The listing builds one solid part. Answer for the finished solid, in the listing's coordinates (mm). Coordinates: 2 decimals unless noted, no trailing zeros. Order: outer loops, then holes, each group sorted by start corner. A loop starts at its lowest first (then second) coordinate and runs counter-clockwise, first axis right, second up. Notation, with made-up numbers: (9.5, 8.5) -> (47.5, 8.5) arc R35 cw to (47.5, 47.5) -> close; hole circle Ø9 at (81.5, -32.5). An arc over 180 degrees is marked (long way). Answer in a Markdown table with one row per item. Add a question column.
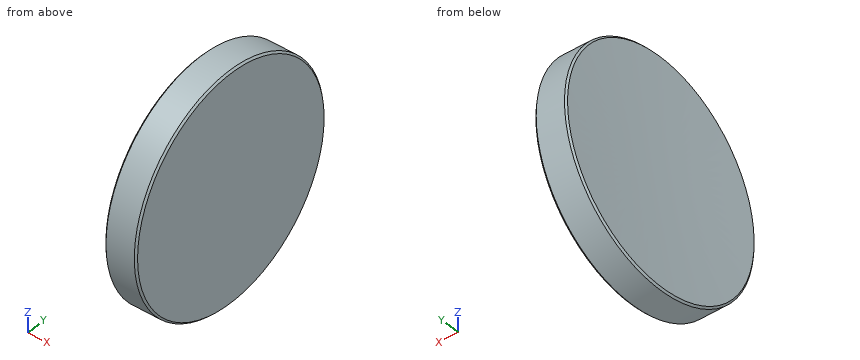
```python
from build123d import *

# Parameters (mm, degrees)
CHAMFER_1_SIZE2       = 0.25
CHAMFER_1_SIZE        = 0.237681877
CHAMFER_1_EDGE_2_SIZE = 0.25


with BuildPart() as part:
    # Эскиз1 → Повернуть1 (revolve)
    with BuildSketch(Plane.XY):
        with BuildLine():
            Line((-0.426259063, 16), (4, 16))
            Line((4, 16), (4, 0))
            Line((4, 0), (0, 0))
            ThreePointArc((0, 0), (-0.106583668, 8.002838509), (-0.426259063, 16))
        make_face()
    revolve(axis=Axis((4, 0, 0), (-1, 0, 0)))

    # Фаска1
    chamfer_1_edges = [part.edges().sort_by_distance(p)[0] for p in [
        (-0.426259063, -16, 0),
    ]]
    chamfer(chamfer_1_edges, length=CHAMFER_1_SIZE, length2=CHAMFER_1_SIZE2)

    # Фаска1 edge 2
    chamfer_1_edge_2_edges = [part.edges().sort_by_distance(p)[0] for p in [
        (4, -16, 0),
    ]]
    chamfer(chamfer_1_edge_2_edges, length=CHAMFER_1_EDGE_2_SIZE)


solid = part.part
```
Q1. Straight lines are drawn through the part: line 1 (X direction, y = -8, z = 6.5); line 2 (Y direction, x = 1.3, z = -3); line 3 (Y direction, x = 2.8, z = -7.5). For each, find the intervals that lie inside material, in ascending order.
Q2. Given pin 1 (1 mm diameter, centred on x = 2, z = -3.5, fed in from +Y); pin 2 (2 mm diameter, centred on x = 3, z = -11, fed in from +Y); pin 3 (1.5 mm diameter, centred on x = 2.5, y = -11, fed in from +Z), each flat-ended and moving along its own axis, determine where each tip first touches the part or whether it passes through.
Q3. A cutting plane is placed at A-A (x = 0.6). Determine the outline of the cut face in (y, z), then the cut area to 3 significant figures.
Returned:
| question | item | result |
|---|---|---|
| 1 | line 1 | x = -0.18 to 4 |
| 1 | line 2 | y = -15.72 to 15.72 |
| 1 | line 3 | y = -14.13 to 14.13 |
| 2 | pin 1 | stops at y = 15.72 |
| 2 | pin 2 | stops at y = 12.49 |
| 2 | pin 3 | stops at z = 12.29 |
| 3 | outline | circle Ø32 at (0, 0) |
| 3 | area | 804 mm² |
